Geometry check sheet. Reference: the model listing, model coordinates, mm. Face numbers are marked on the shaded views. A direction names the side the tool comes from. Give positions to 0.01 mm unless a question says otherwise; leave off trailing zeros. Order: outer loops, then holes, each group sorted by start corner. A loop starts at its lowest first (then second) coordinate and runs counter-clockwise, first axis right, second up. Notation, with made-up numbers: M 6.25,68.25 L 35.25,68.25 A30 cw 35.25,102.25 Z; hole C -10.75,13 d4. An arc over 180 degrees is marked long. Answer as CSV lines item,"result".
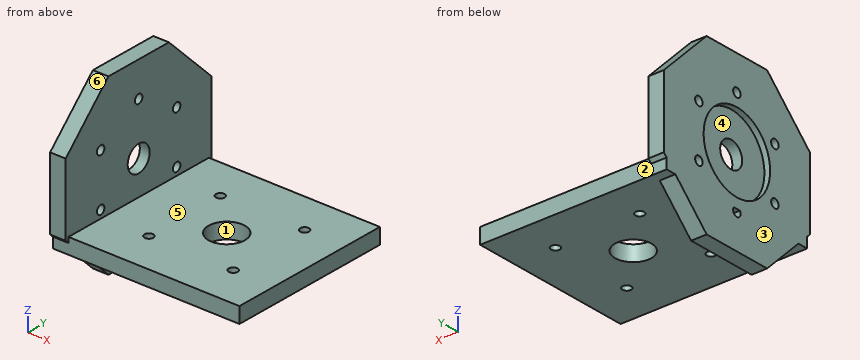
from build123d import *

# Parameters (mm, degrees)
SK_ROLL_PLATE_R         = 1.7
SK_ROLL_PLATE_R_2       = 5
ROLL_PLATE_DEPTH        = 6
SK_YAW_PLATE_W          = 72
SK_YAW_PLATE_H          = 64
SK_YAW_PLATE_R          = 1.7
SK_YAW_PLATE_R_2        = 7
YAW_PLATE_DEPTH         = 6
SK_ROLL_PILOT_RECESS_R  = 15.15
ROLL_PILOT_RECESS_DEPTH = 2.2


with BuildPart() as part:
    # SK_Roll_Plate → Roll_Plate (new body)
    with BuildSketch(Plane(origin=(-40, 0, 0), x_dir=(0, 0, -1), z_dir=(1, 0, 0))):
        Polygon((-13.776603565, -33.25966317), (-33.25966317, -13.776603565), (-33.25966317, 13.776603565), (-13.776603565, 33.25966317), (13.776603565, 33.25966317), (33.25966317, 13.776603565), (33.25966317, -13.776603565), (13.776603565, -33.25966317), align=None)
        with Locations((20, 0)):
            Circle(SK_ROLL_PLATE_R, mode=Mode.SUBTRACT)
        with Locations((10, -17.320508076)):
            Circle(SK_ROLL_PLATE_R, mode=Mode.SUBTRACT)
        with Locations((-10, -17.320508076)):
            Circle(SK_ROLL_PLATE_R, mode=Mode.SUBTRACT)
        with Locations((-20, 0)):
            Circle(SK_ROLL_PLATE_R, mode=Mode.SUBTRACT)
        with Locations((-10, 17.320508076)):
            Circle(SK_ROLL_PLATE_R, mode=Mode.SUBTRACT)
        with Locations((10, 17.320508076)):
            Circle(SK_ROLL_PLATE_R, mode=Mode.SUBTRACT)
        Circle(SK_ROLL_PLATE_R_2, mode=Mode.SUBTRACT)
    extrude(amount=ROLL_PLATE_DEPTH)

    # SK_Yaw_Plate → Yaw_Plate (add)
    with BuildSketch(Plane.XY.offset(-19)):
        with Locations((-4, 0)):
            Rectangle(SK_YAW_PLATE_W, SK_YAW_PLATE_H)
        with Locations((16.263455967, -16.263455967)):
            Circle(SK_YAW_PLATE_R, mode=Mode.SUBTRACT)
        with Locations((-16.263455967, -16.263455967)):
            Circle(SK_YAW_PLATE_R, mode=Mode.SUBTRACT)
        with Locations((-16.263455967, 16.263455967)):
            Circle(SK_YAW_PLATE_R, mode=Mode.SUBTRACT)
        with Locations((16.263455967, 16.263455967)):
            Circle(SK_YAW_PLATE_R, mode=Mode.SUBTRACT)
        Circle(SK_YAW_PLATE_R_2, mode=Mode.SUBTRACT)
    extrude(amount=YAW_PLATE_DEPTH)

    # SK_Roll_Pilot_Recess → Roll_Pilot_Recess (cut)
    with BuildSketch(Plane(origin=(-40, 0, 0), x_dir=(0, 0, -1), z_dir=(1, 0, 0))):
        Circle(SK_ROLL_PILOT_RECESS_R)
    extrude(amount=ROLL_PILOT_RECESS_DEPTH, mode=Mode.SUBTRACT)


solid = part.part
(1) Section check D-D on y = 10.5. Enter the section's corners in (x, z), then the cut area to 3 significant figures.
The answers:
outline,"M -40,-33.26 L -34,-33.26 L -34,-19 L 32,-19 L 32,-13 L -34,-13 L -34,33.26 L -40,33.26 L -40,10.92 L -37.8,10.92 L -37.8,-10.92 L -40,-10.92 Z"
area,"747 mm2"
(2) Section check B-B on z = 10. Enter the section's corners in (x, y), then the cut area to 3 significant figures.
The answers:
outline,"M -40,-33.26 L -34,-33.26 L -34,-19.02 L -40,-19.02 Z; M -40,-15.62 L -34,-15.62 L -34,15.62 L -40,15.62 L -40,11.38 L -37.8,11.38 L -37.8,-11.38 L -40,-11.38 Z; M -40,19.02 L -34,19.02 L -34,33.26 L -40,33.26 Z"
area,"308 mm2"
(3) Material ranges on line 1 (Y direction, x = 0, z = -17); line 2 (X direction, y = 3, z = 19.5); line 3 (Y direction, x = -38, z = 0), recorded low to high.
The answers:
line 1,"y = -32 to -7, 7 to 32"
line 2,"x = -40 to -34"
line 3,"y = -33.26 to -15.15, 15.15 to 33.26"
(4) Section check A-A on x = 0. Enter the section's corners in (y, z), then the cut area to 3 significant figures.
The answers:
outline,"M -32,-19 L -7,-19 L -7,-13 L -32,-13 Z; M 7,-19 L 32,-19 L 32,-13 L 7,-13 Z"
area,"300 mm2"
(5) Draft check along Y on the marked faces 1, 2, 3 and 4. Enter one of: +Y half, -Y half, draft (parallel to the pull), parting line (faces both ways), or undercut.
The answers:
face 1,"undercut"
face 2,"+Y half"
face 3,"draft"
face 4,"undercut"
(6) Tool access check on the marked faces 5 and 6. Record the directions out of +Z, -Z, +X, -X, +Y, -Y that give a thin tool (end or side, any length) a straight path to the whole face; none if there is none.
The answers:
face 5,"+Z, +X, +Y, -Y"
face 6,"+Z, +X, -X, -Y"
(7) Section check C-C on z = -1.5. Enter the section's corners in (x, y).
The answers:
outline,"M -40,-33.26 L -34,-33.26 L -34,-4.77 L -37.8,-4.77 L -37.8,-15.08 L -40,-15.08 Z; M -40,15.08 L -37.8,15.08 L -37.8,4.77 L -34,4.77 L -34,33.26 L -40,33.26 Z"
(8) Gauge pin test, flat ends, axial feed: P1, Ø1.5, axis at x = -9.5, y = -4.5, coming from the -Z side; P2, Ø10, axis at y = -20.5, z = 18.5, coming from the +X side; P3, Ø3, axis at x = -14.5, z = -16.5, coming from the -Y side. Record the tip position at first contact, or that the pin passes through.
The answers:
P1,"stops at z = -19"
P2,"stops at x = -34"
P3,"stops at y = -32"
